from build123d import *

# Parameters (mm, degrees)
F0_W     = 66.9010188431
F0_H     = 36.4210186526
F1_DEPTH = 25.4
F2_R     = 5.08
F3_R     = 5.08
F4_R     = 5.08
F5_R     = 5.08
F6_R     = 5.08
F7_T     = 5.08
F9_D     = 6.35


# Not quite as in the source:
# - a shell that OpenCascade refuses in one call is made with other operations: the cavity is built on its own and cut out


with BuildPart() as f1:
    # F0 (on Top) → F1 (new body)
    with BuildSketch(Plane.XY):
        with Locations((6.1347456649, -7.5554237701)):
            Rectangle(F0_W, F0_H)
    extrude(amount=F1_DEPTH)

    # F2
    f2_edges = [f1.edges().sort_by_distance(p)[0] for p in [
        (6.134746, 10.655086, 25.4),
    ]]
    fillet(f2_edges, radius=F2_R)

    # F3
    f3_edges = [f1.edges().sort_by_distance(p)[0] for p in [
        (6.134746, 10.655086, 0),
    ]]
    fillet(f3_edges, radius=F3_R)

    # F4
    f4_edges = [f1.edges().sort_by_distance(p)[0] for p in [
        (6.134746, -25.765933, 25.4),
    ]]
    fillet(f4_edges, radius=F4_R)

    # F5
    f5_edges = [f1.edges().sort_by_distance(p)[0] for p in [
        (6.134746, -25.765933, 0),
    ]]
    fillet(f5_edges, radius=F5_R)

    # F6
    f6_edges = [f1.edges().sort_by_distance(p)[0] for p in [
        (39.585255, -7.555424, 0),
        (39.585255, 9.167188, 1.487898),
        (39.585255, 9.167188, 23.912102),
        (39.585255, 10.655086, 12.7),
        (39.585255, -7.555424, 25.4),
        (39.585255, -24.278036, 1.487898),
        (39.585255, -25.765933, 12.7),
        (39.585255, -24.278036, 23.912102),
    ]]
    fillet(f6_edges, radius=F6_R)

    # F7: shell of thickness 5.08, made by hand


with BuildPart() as f7_core1:
    # F7_t2: copy of F1
    add(f1.part)

    # the walls: a layer under each face that stays
    f7_faces = [f7_core1.faces().sort_by_distance(p)[0] for p in [
        (39.5852550864, -7.5554237701, 12.7),
        (3.5947456649, -7.5554237701, 0),
        (3.5947456649, -25.7659330964, 12.7),
        (3.5947456649, 10.6550855562, 12.7),
        (3.5947456649, -7.5554237701, 25.4),
    ]]
    thicken(f7_faces, amount=-F7_T, mode=Mode.SUBTRACT)


with BuildPart() as f1_1:
    add(f1.part)

    # what is left inside the walls is the cavity
    f7_cavity = [f7_core1.part.solids().sort_by_distance(p)[0] for p in [
        (3.594746, -11.93226, 5.1308),
    ]]
    add(f7_cavity, mode=Mode.SUBTRACT)

    # F9 (through all)
    with Locations(Plane(origin=(0, 0, 0), x_dir=(1, 0, 0), z_dir=(0, 0, -1))):
        with Locations((-11.171694845, 10.3967795148)):
            Hole(F9_D / 2)


solid = f1_1.part
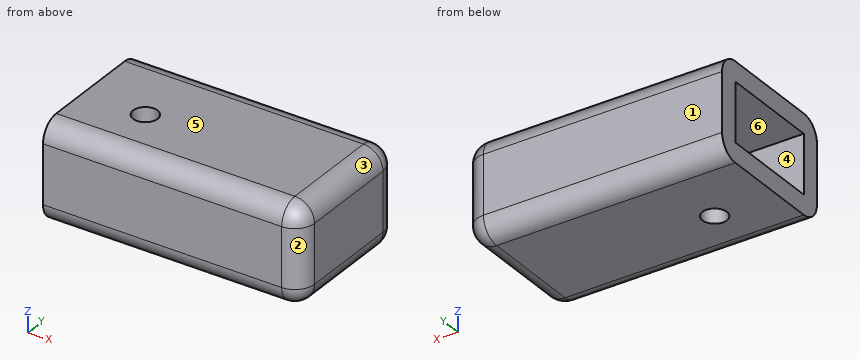
Model file for the job. Use its own axes, mm. Face numbers are marked on the shaded views. A direction names the side the tool comes from. Coordinates: 2 decimals unless noted, no trailing zeros. Order: outer loops, then holes, each group sorted by start corner. A loop starts at its lowest first (then second) coordinate and runs counter-clockwise, first axis right, second up. Notation, with made-up numbers: M 6.25,35 L 24.25,35 A15 cw 24.25,60 Z; hole C 32,49.25 d5. An arc over 180 degrees is marked long. Return JSON: item names as keys, results as strings.
1. Pull direction Y, two halves, no side cores. Call the marked faces 1, 2, 3 and 4: +Y half, -Y half, draft (parallel to the pull), parting line (faces both ways), or undercut.
Ans:
{"face 1": "+Y half", "face 2": "-Y half", "face 3": "draft", "face 4": "undercut"}
2. Tool access for the marked faces 5 and 6: list every direction of +Z, -Z, +X, -X, +Y, -Y with a clear straight run to the whole face (end or side of a thin tool).
Ans:
{"face 5": "+Z, +X, -X, +Y, -Y", "face 6": "-X"}
3. Saw through at A-A (y = -4). Give the cut face in (x, z).
Ans:
{"outline": "M -27.32,0 L 34.51,0 A5.08 ccw 39.59,5.08 L 39.59,20.32 A5.08 ccw 34.51,25.4 L -27.32,25.4 L -27.32,20.32 L 34.51,20.32 L 34.51,5.08 L -27.32,5.08 Z"}
4. Saw through at D-D (z = 7). Give the cut face in (x, y), and give its area (3 significant figures).
Ans:
{"outline": "M -27.32,-25.77 L 34.51,-25.77 A5.08 ccw 39.59,-20.69 L 39.59,5.58 A5.08 ccw 34.51,10.66 L -27.32,10.66 L -27.32,5.58 L 34.51,5.58 L 34.51,-20.69 L -27.32,-20.69 Z", "area": "802 mm^2"}
5. Flat gauge pins, fed straight in: pin 1 (4.5 mm diameter, centred on y = -5.5, z = 16, fed in from -X); pin 2 (1.5 mm diameter, centred on x = -6, z = 22.5, fed in from -Y); pin 3 (2 mm diameter, centred on x = 27, z = 3.5, fed in from +Y). Where does each tip first touch, or does it go through?
Ans:
{"pin 1": "x = 34.51", "pin 2": "y = -25.56", "pin 3": "y = 10.62"}
6. Saw through at C-C (x = -13.5). Give the cut face in (y, z).
Ans:
{"outline": "M -25.77,5.08 A5.08 ccw -20.69,0 L -12.56,0 L -12.56,5.08 L -20.69,5.08 L -20.69,20.32 L -12.56,20.32 L -12.56,25.4 L -20.69,25.4 A5.08 ccw -25.77,20.32 Z; M -8.24,0 L 5.58,0 A5.08 ccw 10.66,5.08 L 10.66,20.32 A5.08 ccw 5.58,25.4 L -8.24,25.4 L -8.24,20.32 L 5.58,20.32 L 5.58,5.08 L -8.24,5.08 Z"}
7. Drill centre lines: probe 1 along Y at (x, z) = (0, 7.25); probe 2 along Z at (x, y) = (-8.5, -2); probe 3 along Z at (x, y) = (22, -21). Where is each one in solid material? Low to high.
Ans:
{"probe 1": "-25.77 to -20.69, 5.58 to 10.66", "probe 2": "0 to 5.08, 20.32 to 25.4", "probe 3": "0.01 to 25.39"}
8. Saw through at B-B (x = 3). Give the cut face in (y, z).
Ans:
{"outline": "M -25.77,5.08 A5.08 ccw -20.69,0 L 5.58,0 A5.08 ccw 10.66,5.08 L 10.66,20.32 A5.08 ccw 5.58,25.4 L -20.69,25.4 A5.08 ccw -25.77,20.32 Z; hole M -20.69,5.08 L 5.58,5.08 L 5.58,20.32 L -20.69,20.32 Z"}
